from build123d import *

# Parameters (mm, degrees)
SKETCH_1_W          = 50
SKETCH_1_H          = 45
EXTRUDE_1_DEPTH     = 8
SKETCH_2_R          = 7.5
EXTRUDE_2_DEPTH     = 50
SKETCH_3_W          = 6
SKETCH_3_H          = 2.5
CUT_EXTRUDE_1_DEPTH = 58
SKETCH_5_R          = 1.5
CUT_EXTRUDE_2_DEPTH = 10


with BuildPart() as part:
    # 草图1 → 凸台-拉伸1 (new body)
    with BuildSketch(Plane.XY):
        Rectangle(SKETCH_1_W, SKETCH_1_H)
    extrude(amount=EXTRUDE_1_DEPTH)

    # 草图2 → 凸台-拉伸2 (add)
    with BuildSketch(Plane(origin=(25, 0, 0), x_dir=(0, 0, -1), z_dir=(1, 0, 0))):
        with BuildLine():
            Line((-8, 10), (-17, 10))
            ThreePointArc((-17, 10), (-27, 0), (-17, -10))
            Line((-17, -10), (-8, -10))
            Line((-8, -10), (-8, 10))
        make_face()
        with Locations((-17, 0)):
            Circle(SKETCH_2_R, mode=Mode.SUBTRACT)
    extrude(amount=-EXTRUDE_2_DEPTH)

    # 草图3 → 切除-拉伸1 (cut)
    with BuildSketch(Plane(origin=(25, 0, 0), x_dir=(0, 0, -1), z_dir=(1, 0, 0))):
        with Locations((-24.5, 0)):
            Rectangle(SKETCH_3_W, SKETCH_3_H)
    extrude(amount=-CUT_EXTRUDE_1_DEPTH, mode=Mode.SUBTRACT)

    # 草图5 → 切除-拉伸2 (cut)
    with BuildSketch(Plane.XY.offset(8)):
        with Locations((-21.5, 19)):
            Circle(SKETCH_5_R)
        with Locations(Location((21.5, 19, 0), (0, 0, 180))):
            Circle(SKETCH_5_R)
        with Locations((21.5, -19)):
            Circle(SKETCH_5_R)
        with Locations(Location((-21.5, -19, 0), (0, 0, 180))):
            Circle(SKETCH_5_R)
    extrude(amount=-CUT_EXTRUDE_2_DEPTH, mode=Mode.SUBTRACT)


solid = part.part
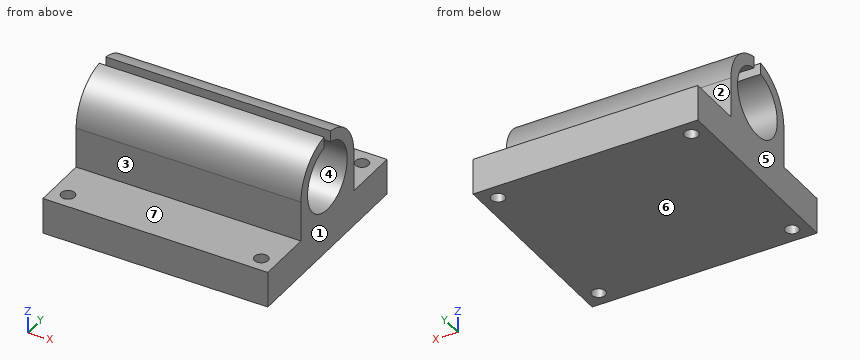
Geometry check sheet. Reference: the model listing, model coordinates, mm. Face numbers are marked on the shaded views. A direction names the side the tool comes from. Round coordinates to 2 decimals unless told otherwise and drop trailing zeros. Order: outer loops, then holes, each group sorted by start corner. A loop starts at its lowest first (then second) coordinate and runs counter-clockwise, first axis right, second up. Notation, with made-up numbers: (16, -26.75) - (27, -26.75) arc R24 cw to (27, -0.75) - close; hole circle Ø2 at (-31, -20). An arc over 180 degrees is marked (long way). One line per question, with ' | ' between items. Start each with the question number.
(1) Depth check by flat-ended pin: pin 1 Ø6 at (x, y) = (-17.5, 15) entering from +Z; pin 2 Ø1.3 at (x, z) = (0.5, 26) entering from +Y; pin 3 Ø2.5 at (x, y) = (-21.5, 19) entering from +Z; pin 4 Ø7 at (x, z) = (-0.5, 14) entering from -Y. Enter the tip coordinate at first touch or a pass-through.
(2) Thickness scan on L1, parallel to Y at x = -21.5, z = 3; L2, parallel to Y at x = -17, z = 16.75; L3, parallel to Z at x = -19.5, y = -15.5. Record the ranges inside material, lowest first. Write a range as [from, to].
(3) Sectioned sample at D-D on y = -3. Record the cut outline in (x, z), and give its area (3 significant figures).
(4) Sectioned sample at B-B on x = -21.5. Record the cut outline in (y, z).
(5) Sectioned sample at C-C on z = 23.5. Record the cut outline in (x, y), and give its area (3 significant figures).
(6) Access from +Z, -Z, +X, -X, +Y, -Y to the whole of each face (thin tool, end or side, straight path). Record for the marked faces 1, 2 and 3.
(7) Release check for a two-part mould opening along Z. For the marked faces 4, 5, 6 and 7 record: released by +Z, released by -Z, zero draft, split by the parting line, or undercut.
(8) Sectioned sample at A-A on y = 19. Record the cut outline in (x, z), and give its area (3 significant figures).
Conclusion:
1) pin 1: stops at z = 8 | pin 2: stops at y = 5.5 | pin 3: passes through | pin 4: stops at y = -10
2) L1: y = [-22.5, -20.5], [-17.5, 17.5], [20.5, 22.5] | L2: y = [-10, -7.5], [7.5, 10] | L3: z = [0, 8]
3) outline: (-25, 0) - (25, 0) - (25, 10.13) - (-25, 10.13) - close; (-25, 23.87) - (25, 23.87) - (25, 26.54) - (-25, 26.54) - close | area: 640 mm2
4) outline: (-22.5, 0) - (-20.5, 0) - (-20.5, 8) - (-22.5, 8) - close; (-17.5, 0) - (17.5, 0) - (17.5, 8) - (10, 8) - (10, 17) arc R10 ccw to (1.25, 26.92) - (1.25, 24.4) arc R7.5 cw (long way) to (-1.25, 24.4) - (-1.25, 26.92) arc R10 ccw to (-10, 17) - (-10, 8) - (-17.5, 8) - close; (20.5, 0) - (22.5, 0) - (22.5, 8) - (20.5, 8) - close
5) outline: (-25, -7.6) - (25, -7.6) - (25, -3.74) - (-25, -3.74) - close; (-25, 3.74) - (25, 3.74) - (25, 7.6) - (-25, 7.6) - close | area: 386 mm2
6) face 1: +Z, -Z, +X, +Y, -Y | face 2: +Z, +X, -X, +Y | face 3: +Z, +X, -X, -Y
7) face 4: undercut | face 5: zero draft | face 6: released by -Z | face 7: released by +Z
8) outline: (-25, 0) - (-23, 0) - (-23, 8) - (-25, 8) - close; (-20, 0) - (20, 0) - (20, 8) - (-20, 8) - close; (23, 0) - (25, 0) - (25, 8) - (23, 8) - close | area: 352 mm2
